from build123d import *

# Parameters (mm, degrees)
SKETCH_1_W          = 186
SKETCH_1_H          = 110
EXTRUDE_1_DEPTH     = 1
SKETCH_2_R          = 1.6
CUT_EXTRUDE_1_DEPTH = 2
EXTRUDE_2_DEPTH     = 1
SKETCH_6_R          = 120
CUT_EXTRUDE_2_DEPTH = 2
SKETCH_8_W          = 186
SKETCH_8_H          = 2
EXTRUDE_3_DEPTH     = 1
SKETCH_7_R          = 1.25
SKETCH_7_R_2        = 1.6
CUT_EXTRUDE_3_DEPTH = 2
CHAMFER_1_SIZE      = 3
FILLET_1_R          = 2
CUT_EXTRUDE_4_DEPTH = 2
SKETCH_10_R         = 1.35
CUT_EXTRUDE_5_DEPTH = 2
SKETCH_11_W         = 12
SKETCH_11_H         = 17.2
CUT_EXTRUDE_6_DEPTH = 2
FILLET_2_R          = 5
FILLET_3_R          = 2


with BuildPart() as part:
    # 草图1 → 凸台-拉伸1 (new body)
    with BuildSketch(Plane(origin=(0, 0, 0), x_dir=(1, 0, 0), z_dir=(0, 1, 0))):
        Rectangle(SKETCH_1_W, SKETCH_1_H)
    extrude(amount=EXTRUDE_1_DEPTH)

    # 草图2 → 切除-拉伸1 (cut, through all)
    with BuildSketch(Plane(origin=(0, 1, 0), x_dir=(1, 0, 0), z_dir=(0, 1, 0))):
        with Locations((90, 15.38)):
            Circle(SKETCH_2_R)
        with Locations((90, 35.38)):
            Circle(SKETCH_2_R)
        with Locations((-90, 35.38)):
            Circle(SKETCH_2_R)
        with Locations((-90, 15.38)):
            Circle(SKETCH_2_R)
    extrude(amount=-CUT_EXTRUDE_1_DEPTH, mode=Mode.SUBTRACT)

    # 草图5 → 凸台-拉伸2 (add)
    with BuildSketch(Plane(origin=(0, 1, 0), x_dir=(1, 0, 0), z_dir=(0, 1, 0))):
        Polygon((-108, -86), (108, -86), (108, -36), (93, -36), (93, -55), (-93, -55), (-93, -36), (-108, -36), align=None)
    extrude(amount=-EXTRUDE_2_DEPTH)

    # 草图6 → 切除-拉伸2 (cut, through all)
    with BuildSketch(Plane(origin=(0, 1, 0), x_dir=(1, 0, 0), z_dir=(0, 1, 0))):
        with Locations((0, -155.12)):
            Circle(SKETCH_6_R)
    extrude(amount=-CUT_EXTRUDE_2_DEPTH, mode=Mode.SUBTRACT)

    # 草图8 → 凸台-拉伸3 (add)
    with BuildSketch(Plane(origin=(0, 1, 0), x_dir=(1, 0, 0), z_dir=(0, 1, 0))):
        with Locations((0, 56)):
            Rectangle(SKETCH_8_W, SKETCH_8_H)
    extrude(amount=-EXTRUDE_3_DEPTH)

    # 草图7 → 切除-拉伸3 (cut, through all)
    with BuildSketch(Plane(origin=(0, 1, 0), x_dir=(1, 0, 0), z_dir=(0, 1, 0))):
        with Locations((47.5, 46.38)):
            Circle(SKETCH_7_R)
        with Locations((47.5, 53.88)):
            Circle(SKETCH_7_R)
        with Locations((102, -74.62)):
            Circle(SKETCH_7_R_2)
        with Locations((102, -54.62)):
            Circle(SKETCH_7_R_2)
        with Locations((-102, -54.62)):
            Circle(SKETCH_7_R_2)
        with Locations((-102, -74.62)):
            Circle(SKETCH_7_R_2)
        with Locations((-47.5, 53.88)):
            Circle(SKETCH_7_R)
        with Locations((-47.5, 46.38)):
            Circle(SKETCH_7_R)
    extrude(amount=-CUT_EXTRUDE_3_DEPTH, mode=Mode.SUBTRACT)

    # 倒角1
    chamfer_1_edges = [part.edges().sort_by_distance(p)[0] for p in [
        (-93, 0.5, 36),
        (93, 0.5, 36),
        (108, 0.5, 36),
        (108, 0.5, 86),
        (-108, 0.5, 86),
        (-108, 0.5, 36),
        (93, 0.5, -57),
        (-93, 0.5, -57),
    ]]
    chamfer(chamfer_1_edges, length=CHAMFER_1_SIZE)

    # 圆角1
    fillet_1_edges = [part.edges().sort_by_distance(p)[0] for p in [
        (-98.093963117, 0.5, 86),
        (98.093963117, 0.5, 86),
    ]]
    fillet(fillet_1_edges, radius=FILLET_1_R)

    # 草图9 → 切除-拉伸4 (cut, through all)
    with BuildSketch(Plane(origin=(0, 1, 0), x_dir=(1, 0, 0), z_dir=(0, 1, 0))):
        with BuildLine():
            Line((16, -29), (-16, -29))
            ThreePointArc((-16, -29), (-17.767766953, -29.732233047), (-18.5, -31.5))
            Line((-18.5, -31.5), (-18.5, -36.554617194))
            ThreePointArc((-18.5, -36.554617194), (0, -35.12), (18.5, -36.554617194))
            Line((18.5, -36.554617194), (18.5, -31.5))
            ThreePointArc((18.5, -31.5), (17.767766953, -29.732233047), (16, -29))
        make_face()
    extrude(amount=-CUT_EXTRUDE_4_DEPTH, mode=Mode.SUBTRACT)

    # 草图10 → 切除-拉伸5 (cut, through all)
    with BuildSketch(Plane(origin=(0, 1, 0), x_dir=(1, 0, 0), z_dir=(0, 1, 0))):
        with Locations((-33.75, -9)):
            Circle(SKETCH_10_R)
        with Locations((-22, 47)):
            Circle(SKETCH_10_R)
        with Locations((22, 47)):
            Circle(SKETCH_10_R)
        with Locations((33.75, -9)):
            Circle(SKETCH_10_R)
        with Locations((41.75, -9)):
            Circle(SKETCH_10_R)
        with Locations((-41.75, -9)):
            Circle(SKETCH_10_R)
        with Locations((41.75, 47)):
            Circle(SKETCH_10_R)
        with Locations((-41.75, 47)):
            Circle(SKETCH_10_R)
    extrude(amount=-CUT_EXTRUDE_5_DEPTH, mode=Mode.SUBTRACT)

    # 草图11 → 切除-拉伸6 (cut, through all)
    with BuildSketch(Plane(origin=(0, 1, 0), x_dir=(1, 0, 0), z_dir=(0, 1, 0))):
        with Locations((0, 48.4)):
            Rectangle(SKETCH_11_W, SKETCH_11_H)
    extrude(amount=-CUT_EXTRUDE_6_DEPTH, mode=Mode.SUBTRACT)

    # 圆角2
    fillet_2_edges = [part.edges().sort_by_distance(p)[0] for p in [
        (6, 0.5, -39.8),
        (-6, 0.5, -39.8),
        (-6, 0.5, -57),
        (6, 0.5, -57),
    ]]
    fillet(fillet_2_edges, radius=FILLET_2_R)

    # 圆角3
    fillet_3_edges = [part.edges().sort_by_distance(p)[0] for p in [
        (18.5, 0.5, 36.554617194),
        (-18.5, 0.5, 36.554617194),
    ]]
    fillet(fillet_3_edges, radius=FILLET_3_R)


solid = part.part
Part model, mm, in its own coordinate system. A direction names the side the tool comes from. Give positions to 0.01 mm unless a question says otherwise; leave off trailing zeros. Loops run counter-clockwise (first coordinate to the right, second up) from the corner with the lowest first, then second, coordinate; pieces in that order, holes last. Notation, with made-up numbers: M 15,71.25 L 20,71.25 A12 cw 20,87.25 Z; hole C -23.5,-13 d10. An arc over 180 degrees is marked long. Put each result on its own line as item: value. Start each with the question number.
1) Probe probe 1 along Z at (x, y) = (-102, 0.45); probe 2 along Z at (x, y) = (-47.5, 0.35); probe 3 along X at (y, z) = (0.5, -53.88). List the from-to ranges inside material, lowest first.
2) 3-axis set-ups, long thin cutter, end or side, ignore diameter. For faces 1 (the flat face through (-2, 0, -2)), 2 (the cylindrical face through (-4.57, 0.49, -41.3)): which of +Z, -Z, +X, -X, +Y, -Y reach the whole face in a straight line?
3) Saw through at C-C (x = 80). List the corners of the cut face in (y, z).
4) Saw through at B-B (z = 25.5). List the corners of the cut face in (x, y), then the cut area to 3 significant figures.
5) Pull direction X, two halves, no side cores. Call faces 3 (the flat face through (-2, 1, -2)), 4 (the cylindrical face through (64.158, 0.507, 53.711)), 5 (the cylindrical face through (-63.05, 0.51, 53.02)): +X half, -X half, draft (parallel to the pull), parting line (faces both ways), or undercut.
6) Saw through at A-A (y = 0.85). State how many separate pieces and enclosed holes the cut face has, then the cut area to 3 significant figures.
Numbers:
1. probe 1: 36 to 53.02, 56.22 to 73.02, 76.22 to 86
1. probe 2: -57 to -55.13, -52.63 to -47.63, -45.13 to 44.92
1. probe 3: -93 to -48.75, -46.25 to -6.37, 6.37 to 46.25, 48.75 to 93
2. face 1: +Z, -Z, +X, -X, -Y
2. face 2: -Z, +Y, -Y
3. outline: M 0,-57 L 1,-57 L 1,65.68 L 0,65.68 Z
4. outline: M -93,0 L 93,0 L 93,1 L -93,1 Z
4. area: 186 mm^2
5. face 3: draft
5. face 4: undercut
5. face 5: undercut
6. separate pieces: 1
6. enclosed holes: 20
6. area: 20,500 mm^2
